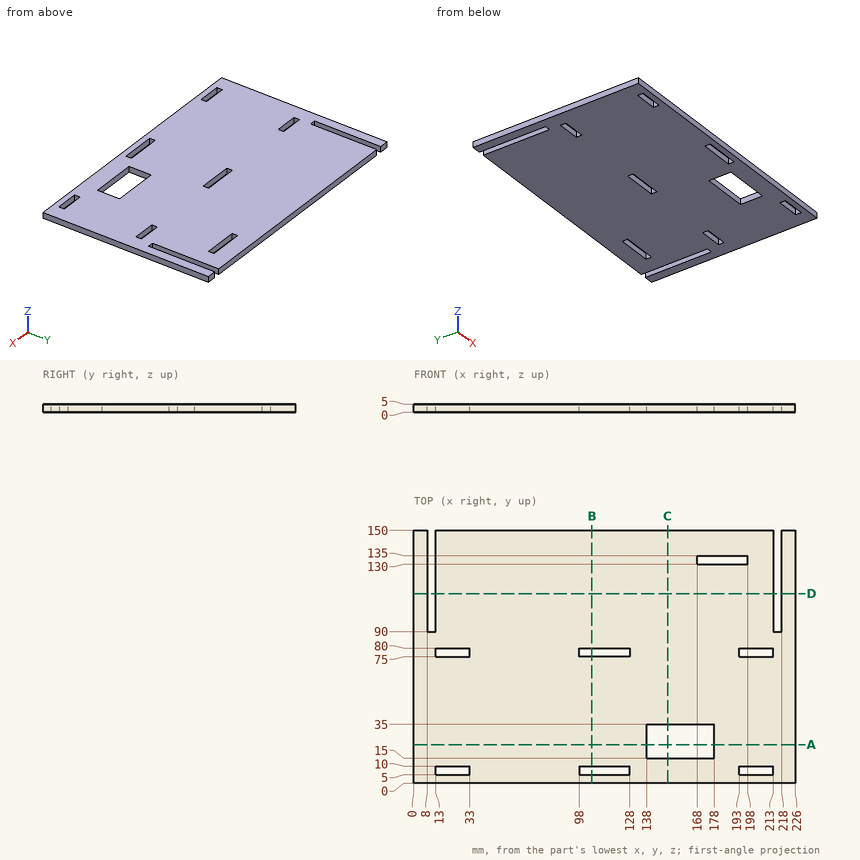
Source: three-view drawing plus pictorial views. Frame: mm from the lowest corner of the part. Round coordinates to 2 decimals unless told otherwise and drop trailing zeros. Loops run counter-clockwise (first coordinate to the right, second up) from the corner with the lowest first, then second, coordinate; pieces in that order, holes last. Notation, with made-up numbers: M -33.75,17 L 21.25,17 A26 cw 21.25,47 Z; hole C 22,63.5 d7. An arc over 180 degrees is marked long. Put each result on its own line as item: value. Start each with the question number.
(1) Section query C-C (x = 150.5). Return loops of the section in (y, z).
(2) Material intervals for line 1 along X through (y, z) = (95, 0.2); line 2 along X through (y, z) = (132, 0.65); line 3 along Y through (x, z) = (211.5, 4.75), sorted ascending. Write a range as [from, to].
(3) Section query D-D (y = 112.5). Return loops of the section in (x, z), then the cut area to 3 significant figures.
(4) Section query B-B (x = 105.5). Return loops of the section in (y, z).
(5) Section query A-A (y = 23). Return loops of the section in (x, z).
Findings below:
1. outline: M 0,0 L 15,0 L 15,5 L 0,5 Z; M 35,0 L 150,0 L 150,5 L 35,5 Z
2. line 1: x = [0, 8], [13, 213], [218, 226]
2. line 2: x = [0, 8], [13, 168], [198, 213], [218, 226]
2. line 3: y = [0, 5], [10, 75], [80, 150]
3. outline: M 0,0 L 8,0 L 8,5 L 0,5 Z; M 13,0 L 213,0 L 213,5 L 13,5 Z; M 218,0 L 226,0 L 226,5 L 218,5 Z
3. area: 1,080 mm2
4. outline: M 0,0 L 5,0 L 5,5 L 0,5 Z; M 10,0 L 75,0 L 75,5 L 10,5 Z; M 80,0 L 150,0 L 150,5 L 80,5 Z
5. outline: M 0,0 L 138,0 L 138,5 L 0,5 Z; M 178,0 L 226,0 L 226,5 L 178,5 Z
